```python
from build123d import *

# Parameters (mm, degrees)
BOSS_EXTRUDE2_DEPTH     = 50.8
CUT_EXTRUDE1_DEPTH      = 103.966915196
CUT_EXTRUDE1_DEPTH_BACK = 103.966915196
FILLET1_R               = 10
FILLET2_R               = 10
FILLET3_R               = 5


with BuildPart() as part:
    # Sketch2 → Boss-Extrude2 (new body)
    with BuildSketch(Plane(origin=(0, 0, 0), x_dir=(1, 0, 0), z_dir=(0, 1, 0))):
        Polygon((0, -10), (0, 10), (60.325, 10), (60.325, -66.2), (41.275, -66.2), (41.275, -10), align=None)
    extrude(amount=BOSS_EXTRUDE2_DEPTH)

    # Sketch3 → Cut-Extrude1 (cut, two sides: drawn at the far end of the back side and taken through both)
    with BuildSketch(Plane.XY.offset(-CUT_EXTRUDE1_DEPTH_BACK)):
        Polygon((12.7, 50.8), (25.4, 6.35), (60.325, 6.35), (60.325, 50.8), align=None)
    extrude(amount=CUT_EXTRUDE1_DEPTH + CUT_EXTRUDE1_DEPTH_BACK, mode=Mode.SUBTRACT)

    # Fillet1
    fillet1_edges = [part.edges().sort_by_distance(p)[0] for p in [
        (25.4, 6.35, 0),
    ]]
    fillet(fillet1_edges, radius=FILLET1_R)

    # Fillet2
    fillet2_edges = [part.edges().sort_by_distance(p)[0] for p in [
        (60.325, 3.175, -10),
        (41.275, 3.175, 10),
    ]]
    fillet(fillet2_edges, radius=FILLET2_R)

    # Fillet3
    fillet3_edges = [part.edges().sort_by_distance(p)[0] for p in [
        (60.325, 3.175, 66.2),
        (41.275, 3.175, 66.2),
    ]]
    fillet(fillet3_edges, radius=FILLET3_R)


solid = part.part
```
The model under review builds one solid part; all positions refer to its coordinate system, in mm. A direction names the side the tool comes from. Round coordinates to 2 decimals unless told otherwise and drop trailing zeros. Loops run counter-clockwise (first coordinate to the right, second up) from the corner with the lowest first, then second, coordinate; pieces in that order, holes last. Notation, with made-up numbers: (-35.5, 64.25) -> (-20.5, 64.25) arc R21 cw to (-20.5, 84.25) -> close; hole circle Ø9 at (73, 43). An arc over 180 degrees is marked (long way). Answer as a JSON object with one key per item and string values. Group by question number.
1) For line 1 (Z direction, x = 14, y = 33); line 2 (Y direction, x = 49.5, z = 39.5), list the stretches that pass through material, from the lowest coordinate up. Write a range as [from, to].
2) Mouldability with a two-part tool opening along Y and no side actions: class faces 1 (the face through (14, 19, -10)), 2 (the face through (26.85, 8.42, 0.21)), 3 (the face through (44, 0, 19)) as released by +Y, released by -Y, zero draft, split by the parting line, or undercut.
3) For faces 4 (the face through (12, 19, 10)), 5 (the face through (51, 3, 66.2)), 6 (the face through (49, 6.35, 28)), list the 3-axis set-ups (+Z, -Z, +X, -X, +Y, -Y) from which the entire face can be reached by the end or side of a thin tool; tool diameter is ignored.
4) We need section D-D on y = 41. Write out the cut boundary in (x, z).
5) We need section C-C on z = -4. Write out the cut boundary in (x, y), then the cut area to 3 significant figures.
6) For pin 1 Ø1.9 at (y, z) = (2, 34.5) entering from -X (3 decimals); pin 2 Ø13.5 at (x, z) = (42, 39) entering from +Y, all flat-tipped, find the tip position at first contact; note any pin that passes through.
7) We need section A-A on y = 3.5. Write out the cut boundary in (x, z) (3 decimals).
8) We need section B-B on x = 14. Write out the cut boundary in (y, z).
Result set:
{
 "1": {"line 1": "[-10, 10]", "line 2": "[0, 6.35]"},
 "2": {"face 1": "zero draft", "face 2": "released by +Y", "face 3": "released by -Y"},
 "3": {"face 4": "+Z, -X, +Y, -Y", "face 5": "+Z, +X, -X, +Y, -Y", "face 6": "+Z, -Z, +X, +Y"},
 "4": {"outline": "(0, -10) -> (15.5, -10) -> (15.5, 10) -> (0, 10) -> close"},
 "5": {"outline": "(0, 0) -> (59.49, 0) -> (59.49, 6.35) -> (32.94, 6.35) arc R10 cw to (23.33, 13.6) -> (12.7, 50.8) -> (0, 50.8) -> close", "area": "1,240 mm²"},
 "6": {"pin 1": "x = 41.275", "pin 2": "y = 6.35"},
 "7": {"outline": "(0, -10) -> (50.325, -10) arc R10 ccw to (60.325, 0) -> (60.325, 61.2) arc R5 ccw to (55.325, 66.2) -> (46.275, 66.2) arc R5 ccw to (41.275, 61.2) -> (41.275, 20) arc R10 cw to (31.275, 10) -> (0, 10) -> close"},
 "8": {"outline": "(0, -10) -> (46.25, -10) -> (46.25, 10) -> (0, 10) -> close"}
}
